Geometry: see drawing. Coordinates: mm, zero at the bounding-box minimum. Give positions to 0.01 mm unless a question says otherwise; leave off trailing zeros. Write each loop counter-clockwise with the first axis right and the second up, starting at its lowest first coordinate (ties: lowest second). Pieces come first, ordered by that corner, then holes. Notation, with made-up numbers: (53.5, -28.5) -> (83.5, -28.5) arc R21 cw to (83.5, -13.5) -> close; hole circle Ø9 at (-19.5, 12). An arc over 180 degrees is marked (long way). Use CSV: the item, a comma, the result in double quotes. Start each with the question number.
1) Section C-C (z = 4.95). Output: boundary loops of the cut face in (x, y).
2) Section D-D (y = 11). Output: boundary loops of the cut face in (x, z).
3) Material intervals for line 1 (X direction, y = 51, z = 1.85) (1 decimal); line 2 (X direction, y = 45.5, z = 5.2); line 3 (Y direction, x = 35, z = 3.05), sorted ascending. Write a range as [from, to].
4) Section B-B (y = 21). Output: boundary loops of the cut face in (x, z).
5) Section A-A (x = 55.5). Output: boundary loops of the cut face in (y, z) (1 decimal).
6) Contact query for flat-ended pins moving along their axis: P1, Ø2, axis at x = 31, z = 3.5, coming from the +Y side; P2, Ø3, axis at y = 38.5, z = 4, coming from the -X side; P3, Ø3.5, axis at x = 73, z = 3.5, coming from the -Y side (1 decimal). Output: stop coordinate, or through.
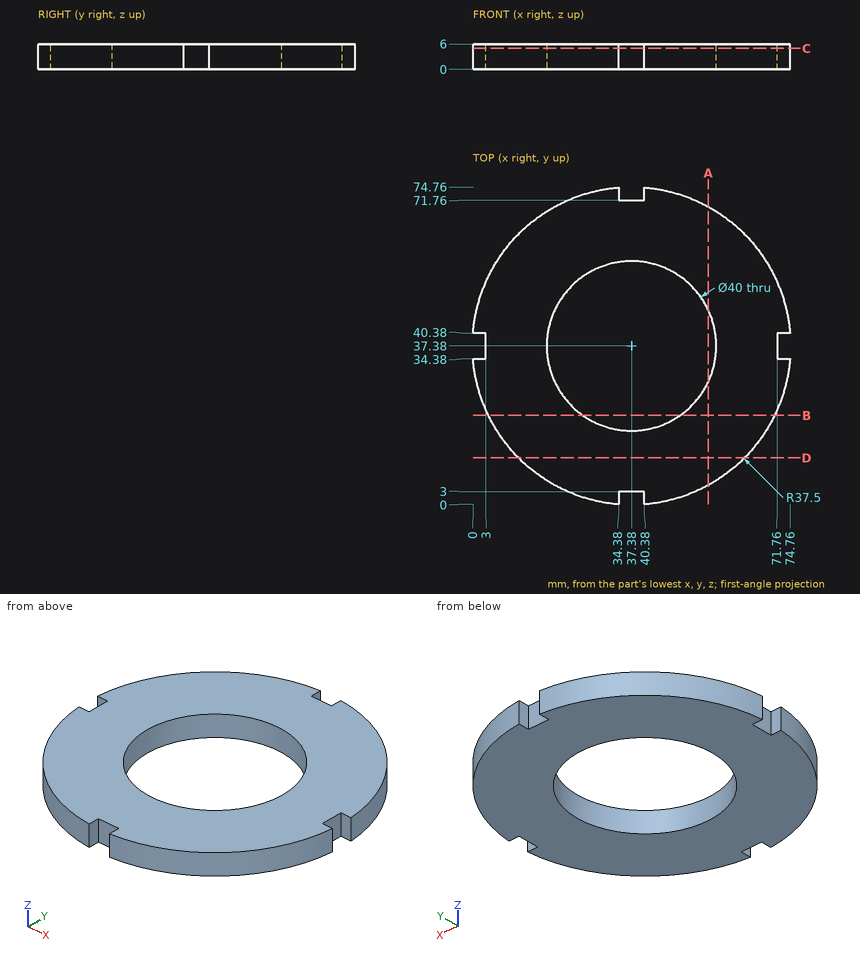
Answers follow:
1,outline,"(0, 34.38) arc R37.5 ccw to (34.38, 0) -> (34.38, 3) -> (40.38, 3) -> (40.38, 0) arc R37.5 ccw to (74.76, 34.38) -> (71.76, 34.38) -> (71.76, 40.38) -> (74.76, 40.38) arc R37.5 ccw to (40.38, 74.76) -> (40.38, 71.76) -> (34.38, 71.76) -> (34.38, 74.76) arc R37.5 ccw to (0, 40.38) -> (3, 40.38) -> (3, 34.38) -> close; hole circle Ø40 at (37.38, 37.38)"
2,outline,"(10.73, 0) -> (64.03, 0) -> (64.03, 6) -> (10.73, 6) -> close"
3,line 1,"x = [2.4, 22.7], [52, 72.3]"
3,line 2,"x = [0.77, 19.1], [55.66, 73.99]"
3,line 3,"y = [3, 17.52], [57.24, 71.76]"
4,outline,"(3.65, 0) -> (25.9, 0) -> (25.9, 6) -> (3.65, 6) -> close; (48.86, 0) -> (71.11, 0) -> (71.11, 6) -> (48.86, 6) -> close"
5,outline,"(4.5, 0) -> (28.9, 0) -> (28.9, 6) -> (4.5, 6) -> close; (45.8, 0) -> (70.2, 0) -> (70.2, 6) -> (45.8, 6) -> close"
6,P1,"stops at y = 74.49"
6,P2,"stops at x = 3"
6,P3,"stops at y = 21.3"
